Input: part model. Units: mm. Frame: model coordinates. Coordinates: 2 decimals unless noted, no trailing zeros. Loops run counter-clockwise (first coordinate to the right, second up) from the corner with the lowest first, then second, coordinate; pieces in that order, holes last. Notation, with made-up numbers: M 67,2 L 91,2 A22 cw 91,33 Z; hole C 59.5,7 d4. An arc over 180 degrees is marked long. Use a Markdown table: item, result. Add a question column.
1. Section B-B on y = 61. Output: boundary loops of the cut face in (x, z), then the cut area to 3 significant figures.
2. Line query: L1, parallel to Y at x = -9.5, z = -2.05; L2, parallel to X at y = 102, z = -2.75; L3, parallel to Y at x = 72.5, z = -1.5. Output: solid intervals per line, ascending. Write a range as [from, to].
3. Pin query (flat end, axial travel): pin 1 (1 mm diameter, centred on x = 9.5, y = 21.81, fed in from -Z); pin 2 (1.5 mm diameter, centred on y = 59, z = -1.5, fed in from +X). Return the tip coordinate at first contact, or that it passes through.
4. Section A-A on z = -1.5. State how many separate pieces and enclosed holes the cut face has, then the cut area to 3 significant figures.
5. Section C-C on y = 91. Output: boundary loops of the cut face in (x, z), then the cut area to 3 significant figures.
```python
from build123d import *

# Parameters (mm, degrees)
BOSS_EXTRUDE1_DEPTH            = 3
F_3_2_3_2_DIAMETER_HOLE1_D     = 3.2
F_3_2_3_2_DIAMETER_HOLE1_DEPTH = 15
F_3_2_3_2_DIAMETER_HOLE1_TIP   = 0.96137699
F_1_6_1_6_DIAMETER_HOLE1_D     = 1.6
F_1_6_1_6_DIAMETER_HOLE1_DEPTH = 15
F_1_6_1_6_DIAMETER_HOLE1_TIP   = 0.480688495


with BuildPart() as part:
    # Sketch1 → Boss-Extrude1 (new body)
    with BuildSketch(Plane.XY):
        with BuildLine():
            Line((-11.618950039, 112.409005395), (11.618950039, 112.409005395))
            Line((11.618950039, 112.409005395), (130.207854482, 112.409005395))
            add(Edge.make_bspline(
                [(134.178039088, 108.917568146), (133.74675554, 112.409005395), (130.207854482, 112.409005395)],
                knots=[0.122173048, 0.122173048, 0.122173048, 1.570796327, 1.570796327, 1.570796327], degree=2, weights=[1, 0.748955721, 1]))
            Line((134.178039088, 108.917568146), (146.527006833, 8.947035697))
            add(Edge.make_bspline(
                [(146.556822227, 8.462484609), (146.556822227, 8.705666473), (146.527006833, 8.947035697)],
                knots=[0, 0, 0, 0.122173048, 0.122173048, 0.122173048], degree=2, weights=[1, 0.998134798, 1]))
            Line((146.556822227, 8.462484609), (146.556822227, -0.579261565))
            add(Edge.make_bspline(
                [(142.556822227, -4.555249901), (146.556822227, -4.555249901), (146.556822227, -0.579261565)],
                knots=[4.71238898, 4.71238898, 4.71238898, 6.283185307, 6.283185307, 6.283185307], degree=2, weights=[1, 0.707106781, 1]))
            Line((142.556822227, -4.555249901), (-142.556822227, -4.555249901))
            add(Edge.make_bspline(
                [(-146.556822227, -0.579261565), (-146.556822227, -4.555249901), (-142.556822227, -4.555249901)],
                knots=[3.141592654, 3.141592654, 3.141592654, 4.71238898, 4.71238898, 4.71238898], degree=2, weights=[1, 0.707106781, 1]))
            Line((-146.556822227, -0.579261565), (-146.556822227, 8.462484609))
            add(Edge.make_bspline(
                [(-146.527006833, 8.947035697), (-146.556822227, 8.705666473), (-146.556822227, 8.462484609)],
                knots=[3.019419606, 3.019419606, 3.019419606, 3.141592654, 3.141592654, 3.141592654], degree=2, weights=[1, 0.998134798, 1]))
            Line((-146.527006833, 8.947035697), (-134.178039088, 108.917568146))
            add(Edge.make_bspline(
                [(-130.207854482, 112.409005395), (-133.74675554, 112.409005395), (-134.178039088, 108.917568146)],
                knots=[1.570796327, 1.570796327, 1.570796327, 3.019419606, 3.019419606, 3.019419606], degree=2, weights=[1, 0.748955721, 1]))
            Line((-130.207854482, 112.409005395), (-11.618950039, 112.409005395))
        make_face()
    extrude(amount=-BOSS_EXTRUDE1_DEPTH)

    # Ø3.2 (3.2) Diameter Hole1
    with Locations(Plane(origin=(167.519332635, 69.709864468, 0), x_dir=(1, 0, 0), z_dir=(0, 0, 1))):
        with Locations((-47.07064809, 39.062428571), (-29.962510408, -70.289126033), (-93.981129185, -69.295128949), (-241.057536085, -69.295128949), (-305.076154862, -70.289126033), (-287.968017181, 39.062428571), (-182.519332635, 33.699140926), (-152.519332635, 33.699140926), (-162.519332635, -70.289126033)):
            Hole(F_3_2_3_2_DIAMETER_HOLE1_D / 2, depth=F_3_2_3_2_DIAMETER_HOLE1_DEPTH)
            with Locations((0, 0, -(F_3_2_3_2_DIAMETER_HOLE1_DEPTH + F_3_2_3_2_DIAMETER_HOLE1_TIP / 2))):  # 118° drill point
                Cone(0, F_3_2_3_2_DIAMETER_HOLE1_D / 2, F_3_2_3_2_DIAMETER_HOLE1_TIP, mode=Mode.SUBTRACT)

    # Ø1.6 (1.6) Diameter Hole1
    with Locations(Plane.XY):
        with Locations((-9.5, 68.809005395), (9.5, 68.809005395), (-9.5, 21.809005395), (9.5, 21.809005395)):
            Hole(F_1_6_1_6_DIAMETER_HOLE1_D / 2, depth=F_1_6_1_6_DIAMETER_HOLE1_DEPTH)
            with Locations((0, 0, -(F_1_6_1_6_DIAMETER_HOLE1_DEPTH + F_1_6_1_6_DIAMETER_HOLE1_TIP / 2))):  # 118° drill point
                Cone(0, F_1_6_1_6_DIAMETER_HOLE1_D / 2, F_1_6_1_6_DIAMETER_HOLE1_TIP, mode=Mode.SUBTRACT)


solid = part.part
```
Answers below:
| question | item | result |
|---|---|---|
| 1 | outline | M -140.1,-3 L 140.1,-3 L 140.1,0 L -140.1,0 Z |
| 1 | area | 841 mm² |
| 2 | L1 | y = [-4.56, 21.01], [22.61, 68.01], [69.61, 112.41] |
| 2 | L2 | x = [-135.03, -15.76], [-14.24, 14.24], [15.76, 135.03] |
| 2 | L3 | y = [-4.56, -0.8], [1.63, 112.41] |
| 3 | pin 1 | passes through |
| 3 | pin 2 | stops at x = 140.44 |
| 4 | separate pieces | 1 |
| 4 | enclosed holes | 13 |
| 4 | area | 32,900 mm² |
| 5 | outline | M -136.39,-3 L 136.39,-3 L 136.39,0 L -136.39,0 Z |
| 5 | area | 818 mm² |
